Answer from the drawing. Dimensions are ordinates in mm from the lowest x, y and z of the part. A direction names the side the tool comes from. Coordinates: 2 decimals unless noted, no trailing zeros. Order: outer loops, then holes, each group sorted by start corner. A loop starts at its lowest first (then second) coordinate and runs counter-clockwise, first axis right, second up. Notation, with made-up numbers: (-16.5, 84) - (22.5, 84) arc R21 ccw to (22.5, 121) - close; hole circle Ø7 at (0, -35.5). An arc over 180 degrees is marked (long way). One line per item, written item: value. Start each with the question number.
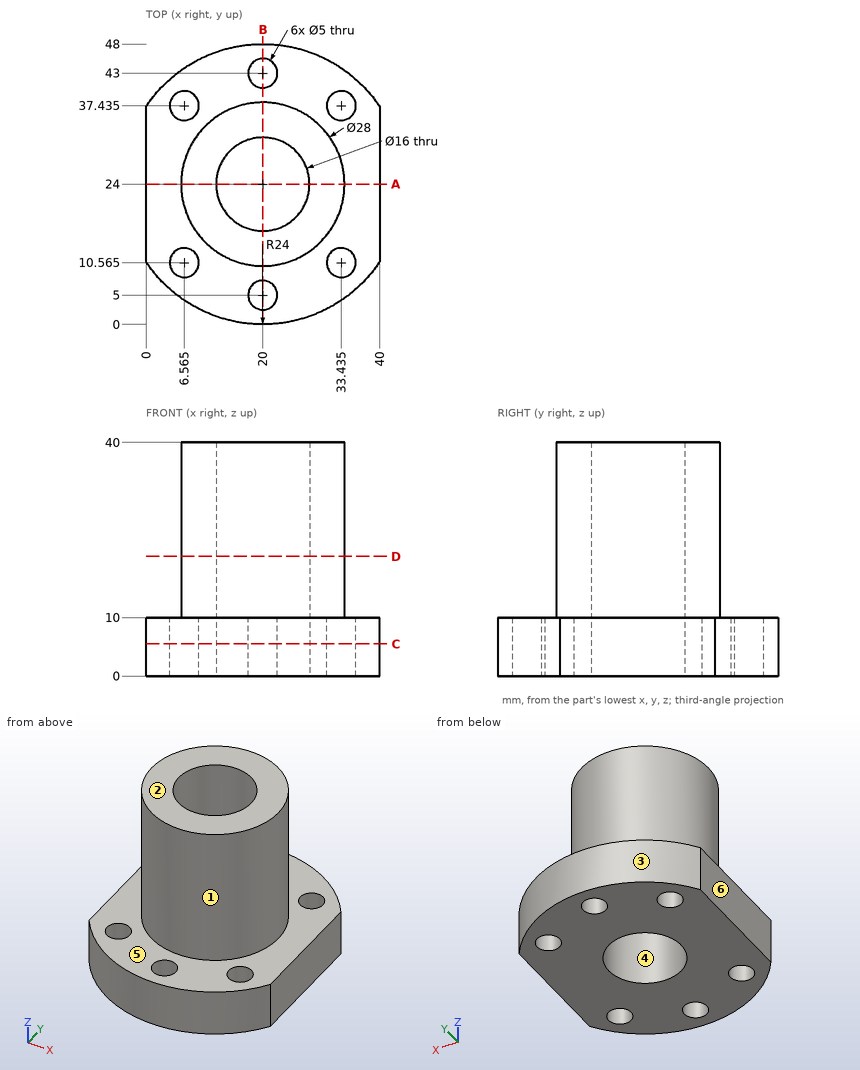
(1) For a pull along X with two mould halves and no side action, classify the marked faces 3, 4, 5 and 6 as pulls with the +X half, pulls with the -X half, needs draft (parallel to the pull), parting line crosses it, or undercut.
(2) The part is cut by section A-A on y = 24. Determine the outline of the cut face in (x, z).
(3) The part is cut by section C-C on z = 5.5. Determine the outline of the cut face in (x, y) (1 decimal).
(4) The part is cut by section B-B on x = 20. Determine the outline of the cut face in (y, z), plus the area to 3 significant figures.
(5) Consider probe 1 along Y at (x, z) = (4.5, 8); probe 2 along Y at (x, z) = (32, 7.5); probe 3 along Y at (x, z) = (20, 25.5). Determine where each line is inside the solid, lowest interval first.
(6) The part is cut by section D-D on z = 20.5. Determine the outline of the cut face in (x, y).
(7) For the marked faces 1 and 2, determine the directions among +Z, -Z, +X, -X, +Y, -Y from which every point of the face is accessible in a straight line to the end or side of a thin tool.
(8) Flat-ended cylindrical pins translate along their axes: pin 1 Ø8 at (x, y) = (6.56, 37.44) entering from +Z; pin 2 Ø6 at (x, z) = (8, 27) entering from -Y; pin 3 Ø3 at (x, z) = (27, 4.5) entering from -Y. Find the tip coordinate at first contact, or state that the pin passes through.
Completed:
1. face 3: parting line crosses it
1. face 4: undercut
1. face 5: needs draft
1. face 6: pulls with the -X half
2. outline: (0, 0) - (12, 0) - (12, 40) - (6, 40) - (6, 10) - (0, 10) - close; (28, 0) - (40, 0) - (40, 10) - (34, 10) - (34, 40) - (28, 40) - close
3. outline: (0, 10.7) arc R24 ccw to (40, 10.7) - (40, 37.3) arc R24 ccw to (0, 37.3) - close; hole circle Ø5 at (6.6, 10.6); hole circle Ø5 at (6.6, 37.4); hole circle Ø16 at (20, 24); hole circle Ø5 at (20, 5); hole circle Ø5 at (20, 43); hole circle Ø5 at (33.4, 10.6); hole circle Ø5 at (33.4, 37.4)
4. outline: (0, 0) - (2.5, 0) - (2.5, 10) - (0, 10) - close; (7.5, 0) - (16, 0) - (16, 40) - (10, 40) - (10, 10) - (7.5, 10) - close; (32, 0) - (40.5, 0) - (40.5, 10) - (38, 10) - (38, 40) - (32, 40) - close; (45.5, 0) - (48, 0) - (48, 10) - (45.5, 10) - close
4. area: 580 mm2
5. probe 1: y = 5.68 to 9.16, 11.97 to 36.03, 38.84 to 42.32
5. probe 2: y = 3.22 to 8.52, 12.61 to 35.39, 39.48 to 44.78
5. probe 3: y = 10 to 16, 32 to 38
6. outline: circle Ø28 at (20, 24); hole circle Ø16 at (20, 24)
7. face 1: +Z
7. face 2: +Z, +X, -X, +Y, -Y
8. pin 1: stops at z = 10
8. pin 2: stops at y = 13.28
8. pin 3: stops at y = 0.64
